Build history of the part. All positions in model axes, mm. Face numbers are marked on the shaded views. A direction names the side the tool comes from. Give positions to 0.01 mm unless a question says otherwise; leave off trailing zeros. Loops run counter-clockwise (first coordinate to the right, second up) from the corner with the lowest first, then second, coordinate; pieces in that order, holes last. Notation, with made-up numbers: (79, 25) -> (91, 25) arc R5 cw to (91, 34) -> close; hole circle Ø9 at (-1.75, 24.25). An arc over 180 degrees is marked (long way). One line per question, with ' | ' between items. Start each with the question number.
(1) Mould opens along X. For the marked faces 6, 7 and 8 say: pulls with the +X half, pulls with the -X half, needs draft (parallel to the pull), parting line crosses it, or undercut.
(2) Slice it at D-D, the plane z = 4. Write the cut outline in (x, y) (3 decimals), then the cut area to 3 significant figures.
(3) Slice it at B-B, the plane y = -32. Write the cut outline in (x, z).
(4) Flat gauge pins, fed straight in: pin 1 Ø15 at (y, z) = (-35, -11) entering from -X; pin 2 Ø8 at (x, y) = (-31.5, -14.5) entering from +Z; pin 3 Ø1 at (x, y) = (-15.5, -38) entering from +Z. Where does each tip first touch, or does it go through?
(5) Drill centre lines: L1, parallel to X at y = -34, z = -16.5; L2, parallel to Z at x = -36.5, y = -52.5; L3, parallel to Y at x = 16, z = -15. Where is each one in solid material? Low to high. Write a range as from..to.
(6) Slice it at A-A, the plane x = 0. Write the cut outline in (y, z).
(7) 3-axis set-ups, long thin cutter, end or side, ignore diameter. For the marked faces 1, 2, 3, 4 and 5: which of +Z, -Z, +X, -X, +Y, -Y reach the whole face in a straight line?
```python
from build123d import *

# Parameters (mm, degrees)
F1_DEPTH  = 2
F2_R      = 1.5
F3_DEPTH  = 5
F4_R      = 19
F5_DEPTH  = 27
F6_W      = 47
F6_H      = 27
F7_DEPTH  = 5
F8_W      = 27
F8_H      = 5
F9_DEPTH  = 20
F10_W     = 27
F10_H     = 5
F11_DEPTH = 20
F12_R     = 4.99999
F14_DEPTH = 30
F16_DEPTH = 4
F18_DEPTH = 25


# Not quite as in the source:
# - a fillet or chamfer is up to 0.001 mm smaller than in the source, because OpenCascade refuses the exact size


with BuildPart() as f1:
    # F0 (on Front) → F1 (new body)
    with BuildSketch(Plane.XZ):
        with BuildLine():
            Line((-23.5, -23.5), (0, -23.5))
            Line((0, -23.5), (23.5, -23.5))
            Line((23.5, -23.5), (23.5, 0))
            ThreePointArc((23.5, 0), (0, 23.5), (-23.5, 0))
            Line((-23.5, 0), (-23.5, -23.5))
        make_face()
    extrude(amount=F1_DEPTH)

    # F2 (on face) → F3 (cut)
    with BuildSketch(Plane.XZ.offset(2)):
        with Locations((15.5, 0)):
            Circle(F2_R)
        with Locations((7.75, 13.4233937587)):
            Circle(F2_R)
        with Locations((-7.75, 13.4233937587)):
            Circle(F2_R)
        with Locations((-15.5, 0)):
            Circle(F2_R)
        with Locations((-7.75, -13.4233937587)):
            Circle(F2_R)
        with Locations((7.75, -13.4233937587)):
            Circle(F2_R)
        with BuildLine():
            Line((6.5, -7), (6.5, 7))
            ThreePointArc((6.5, 7), (0, 13.5), (-6.5, 7))
            Line((-6.5, 7), (-6.5, -7))
            ThreePointArc((-6.5, -7), (0, -13.5), (6.5, -7))
        make_face()
    extrude(amount=-F3_DEPTH, mode=Mode.SUBTRACT)

    # F4 (on Front) → F5 (join)
    with BuildSketch(Plane.XZ):
        with BuildLine():
            ThreePointArc((23.5, 0), (0, 23.5), (-23.5, 0))
            Line((-23.5, 0), (-23.5, -23.5))
            Line((-23.5, -23.5), (23.5, -23.5))
            Line((23.5, -23.5), (23.5, 0))
        make_face()
        with Locations((0, -0.6784388353)):
            Circle(F4_R, mode=Mode.SUBTRACT)
    extrude(amount=F5_DEPTH)

    # F6 (on face) → F7 (join)
    with BuildSketch(Plane(origin=(0, 0, -23.5), x_dir=(1, 0, 0), z_dir=(0, 0, -1))):
        with Locations((0, 13.5)):
            Rectangle(F6_W, F6_H)
    extrude(amount=F7_DEPTH)

    # F8 (on face) → F9 (join)
    with BuildSketch(Plane(origin=(-23.5, 0, 0), x_dir=(0, -1, 0), z_dir=(-1, 0, 0))):
        with Locations((13.5, -26)):
            Rectangle(F8_W, F8_H)
    extrude(amount=F9_DEPTH)

    # F10 (on face) → F11 (join)
    with BuildSketch(Plane.YZ.offset(23.5)):
        with Locations((-13.5, -26)):
            Rectangle(F10_W, F10_H)
    extrude(amount=F11_DEPTH)

    # F12 (radius 5 in the source; OpenCascade refuses exactly that, so slightly less here)
    f12_edges = [f1.edges().sort_by_distance(p)[0] for p in [
        (23.5, -13.5, -23.5),
        (43.5, -13.5, -23.5),
        (-23.5, -13.5, -23.5),
        (-43.5, -13.5, -23.5),
    ]]
    fillet(f12_edges, radius=F12_R)

    # F13 (on face) → F14 (join)
    with BuildSketch(Plane.XZ.offset(27)):
        with BuildLine():
            Line((23.5, -18.5), (23.5, 0))
            ThreePointArc((23.5, 0), (0, 23.5), (-23.5, 0))
            Line((-23.5, 0), (-23.5, -18.5))
            ThreePointArc((-23.5, -18.5), (-24.9644660941, -22.0355339059), (-28.5, -23.5))
            Line((-28.5, -23.5), (-38.5, -23.5))
            ThreePointArc((-38.5, -23.5), (-42.0355339059, -24.9644660941), (-43.5, -28.5))
            Line((-43.5, -28.5), (-19, -28.5))
            Line((-19, -28.5), (-19, -0.6784388353))
            ThreePointArc((-19, -0.6784388353), (0, 18.3215611647), (19, -0.6784388353))
            Line((19, -0.6784388353), (19, -28.5))
            Line((19, -28.5), (43.5, -28.5))
            ThreePointArc((43.5, -28.5), (42.0355339059, -24.9644660941), (38.5, -23.5))
            Line((38.5, -23.5), (28.5, -23.5))
            ThreePointArc((28.5, -23.5), (24.9644660941, -22.0355339059), (23.5, -18.5))
        make_face()
    extrude(amount=F14_DEPTH)

    # F15 (on face) → F16 (join)
    with BuildSketch(Plane.XZ.offset(57)):
        with BuildLine():
            ThreePointArc((6.0827625303, 17.3215611647), (3.0822070015, 18.0698944239), (0, 18.3215611647))
            Line((0, 18.3215611647), (0, 17.3215611647))
            Line((0, 17.3215611647), (6.0827625303, 17.3215611647))
        make_face()
        with BuildLine():
            Line((0, 17.3215611647), (0, 18.3215611647))
            ThreePointArc((0, 18.3215611647), (-3.0822070015, 18.0698944239), (-6.0827625303, 17.3215611647))
            Line((-6.0827625303, 17.3215611647), (0, 17.3215611647))
        make_face()
    extrude(amount=-F16_DEPTH)

    # F17 (on face) → F18 (cut)
    with BuildSketch(Plane(origin=(0, 0, -28.5), x_dir=(1, 0, 0), z_dir=(0, 0, -1))):
        with BuildLine():
            ThreePointArc((-35, 5.5), (-34.5606601718, 4.4393398282), (-33.5, 4))
            Line((-33.5, 4), (-33.5, 5.5))
            Line((-33.5, 5.5), (-35, 5.5))
        make_face()
        with BuildLine():
            ThreePointArc((35, 51.5), (33.5, 53), (32, 51.5))
            ThreePointArc((32, 51.5), (33.5, 50), (35, 51.5))
        make_face()
        with BuildLine():
            ThreePointArc((-33.5, 53), (-35, 51.5), (-33.5, 50))
            Line((-33.5, 50), (-33.5, 51.5))
            Line((-33.5, 51.5), (-33.5, 53))
        make_face()
        with BuildLine():
            Line((-33.5, 51.5), (-33.5, 50))
            ThreePointArc((-33.5, 50), (-32.4393398282, 50.4393398282), (-32, 51.5))
            Line((-32, 51.5), (-33.5, 51.5))
        make_face()
        with BuildLine():
            ThreePointArc((35, 5.5), (33.5, 7), (32, 5.5))
            ThreePointArc((32, 5.5), (33.5, 4), (35, 5.5))
        make_face()
        with BuildLine():
            Line((-33.5, 5.5), (-33.5, 4))
            ThreePointArc((-33.5, 4), (-32.4393398282, 4.4393398282), (-32, 5.5))
            Line((-32, 5.5), (-33.5, 5.5))
        make_face()
        with BuildLine():
            Line((-33.5, 7), (-33.5, 5.5))
            Line((-33.5, 5.5), (-32, 5.5))
            ThreePointArc((-32, 5.5), (-32.4393398282, 6.5606601718), (-33.5, 7))
        make_face()
        with BuildLine():
            Line((-35, 5.5), (-33.5, 5.5))
            Line((-33.5, 5.5), (-33.5, 7))
            ThreePointArc((-33.5, 7), (-34.5606601718, 6.5606601718), (-35, 5.5))
        make_face()
        with BuildLine():
            ThreePointArc((-32, 51.5), (-32.4393398282, 52.5606601718), (-33.5, 53))
            Line((-33.5, 53), (-33.5, 51.5))
            Line((-33.5, 51.5), (-32, 51.5))
        make_face()
    extrude(amount=-F18_DEPTH, mode=Mode.SUBTRACT)


solid = f1.part
```
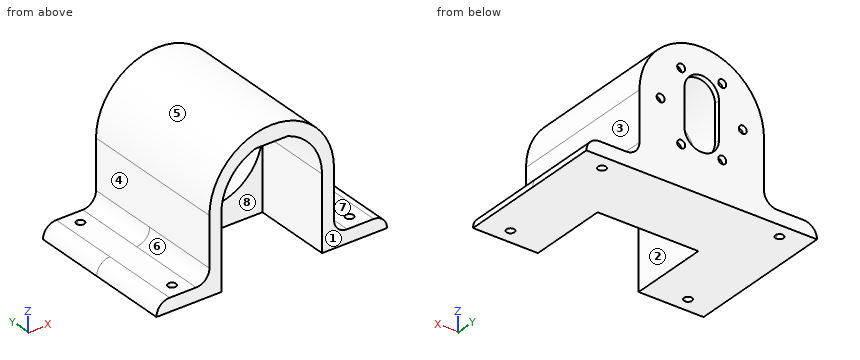
Final values:
1) face 6: pulls with the -X half | face 7: needs draft | face 8: undercut
2) outline: (-23.157, -57) -> (-18.415, -57) -> (-18.415, -2) -> (-6.5, -2) -> (-6.5, 0) -> (-23.157, 0) -> close; (6.5, -2) -> (18.415, -2) -> (18.415, -57) -> (23.157, -57) -> (23.157, 0) -> (6.5, 0) -> close | area: 588 mm2
3) outline: (-43.5, -28.5) -> (-19, -28.5) -> (-19, -0.68) arc R19 cw to (19, -0.68) -> (19, -28.5) -> (43.5, -28.5) arc R5 ccw to (38.5, -23.5) -> (28.5, -23.5) arc R5 cw to (23.5, -18.5) -> (23.5, 0) arc R23.5 ccw to (-23.5, 0) -> (-23.5, -18.5) arc R5 cw to (-28.5, -23.5) -> (-38.5, -23.5) arc R5 ccw to start
4) pin 1: x = -23.5 | pin 2: z = -23.4 | pin 3: z = 18.09
5) L1: -23.5..-19, 19..23.5 | L2: -28.5..-23.5 | L3: -27..0
6) outline: (-57, 17.32) -> (-53, 17.32) -> (-53, 18.32) -> (-2, 18.32) -> (-2, 13.5) -> (0, 13.5) -> (0, 23.5) -> (-57, 23.5) -> close; (-27, -28.5) -> (0, -28.5) -> (0, -13.5) -> (-2, -13.5) -> (-2, -19.68) -> (-27, -19.68) -> close
7) face 1: +Z, -Z, +X, -X, -Y | face 2: -Z, -Y | face 3: +Z, +X, +Y, -Y | face 4: +Z, -X, +Y, -Y | face 5: +Z, +Y, -Y
